Autodesk Inventor part; units mm, degrees
ref_plane "nt_XY" through (0, 0, 0) normal (1, 0, 0) x (0, 0, -1)
ref_plane "nt_YZ" through (0, 0, 0) normal (0, 0, -1) x (0, 1, 0)
ref_plane "nt_ZX" through (0, 0, 0) normal (0, 1, 0) x (1, 0, 0)
sketch "B" plane through (0, 0, 0) normal (1, 0, 0) x (0, 1, 0)
  line L0 (-3.1754, 5.5) -> (-6.3509, 0)
  line L1 (-6.3509, 0) -> (-3.1754, -5.5)
  line L2 (-3.1754, -5.5) -> (3.1754, -5.5)
  line L3 (3.1754, -5.5) -> (6.3509, 0)
  line L4 (6.3509, 0) -> (3.1754, 5.5)
  line L5 (3.1754, 5.5) -> (-3.1754, 5.5)
extrude "Extrusion1" add sketch "B" along normal mid plane 4
sketch "Sketch_2_ALT_Drilling_1" plane through (0, 0, 0) normal (0, 0, 1) x (1, 0, 0)
  line L0 (2, 0) -> (-2, 0)
  line L1 (-2, 0) -> (-2, 4)
  line L2 (-2, 4) -> (-1.4585, 3.4585)
  line L3 (-1.4585, 3.4585) -> (1.4585, 3.4585)
  line L4 (1.4585, 3.4585) -> (2, 4)
  line L5 (2, 4) -> (2, 0)
  line L6 (2, 0) -> (-2, 0)
revolve "Revolution1" cut sketch "Sketch_2_ALT_Drilling_1" angle 360 about axis through (2, 0, 0) along (1, 0, 0)
thread "Thread1"
sketch "Sketch_3" plane through (0, 0, 0) normal (0, 0, 1) x (1, 0, 0)
  line L0 (50, 0) -> (-50, 0)
  line L1 (-7, 1) -> (-2, 1)
  line L2 (-2, 1) -> (-2, 5.5)
  line L3 (-2, 5.5) -> (0, 8.9641)
  line L4 (0, 8.9641) -> (2, 5.5)
  line L5 (2, 5.5) -> (2, 1)
  line L6 (2, 1) -> (7, 1)
  line L7 (7, 1) -> (7, 13.5)
  line L8 (7, 13.5) -> (-7, 13.5)
  line L9 (-7, 13.5) -> (-7, 1)
revolve "Revolution2" cut sketch "Sketch_3" angle 360 about axis through (50, 0, 0) along (1, 0, 0)
ref_plane "nt_XY" through (0, 0, 0) normal (1, 0, 0) x (0, 0, -1)
ref_plane "nt_YZ" through (0, 0, 0) normal (0, 0, -1) x (0, 1, 0)
ref_plane "nt_ZX" through (0, 0, 0) normal (0, 1, 0) x (1, 0, 0)
ref_plane "ntj_XY" through (2, 0, 0) normal (1, 0, 0) x (0, 0, -1)
ref_plane "ntj_YZ" through (2, 0, 0) normal (0, 0, -1) x (0, 1, 0)
ref_plane "ntj_ZX" through (2, 0, 0) normal (0, 1, 0) x (1, 0, 0)
properties part number "SNJ-010C"
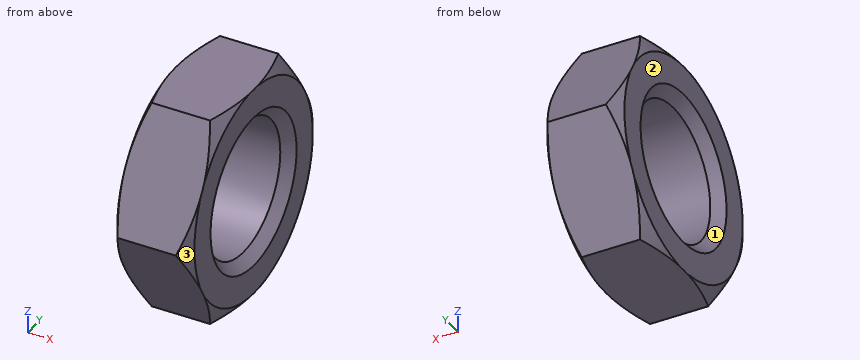
Can you work these out from the model? Positions are in its coordinate system, mm. Face numbers are marked on the shaded views. Round coordinates to 2 decimals unless told otherwise and drop trailing zeros. Order: outer loops, then holes, each group sorted by start corner. A loop starts at its lowest first (then second) coordinate and runs counter-clockwise, first axis right, second up. Notation, with made-up numbers: (26.5, -18.5) -> (38.5, -18.5) arc R22 cw to (38.5, 16.5) -> close; hole circle Ø9 at (3, 38). An arc over 180 degrees is marked (long way). Write each question's results on one line, items separated by ' | '. Start each with the question number.
Item 1: If we section it at A-A, the plane x = 0.45: Write out the boundary of the cut face in (y, z).
Item 2: Please list where these lines run through material, in increasing order: L1, parallel to Z at x = 0.2, y = 0; L2, parallel to Z at x = 0.25, y = -2; L3, parallel to Y at x = 1.7, z = 2.
Item 3: Thinking about a two-plate mould opening in Y: for the marked faces 1, 2 and 3, which applies, +Y half, -Y half, draft (parallel to the pull), parting line (faces both ways), or undercut?
Item 4: Will these pins go through, and if not, where does the flat tip stop? pin 1 (2 mm diameter, centred on x = -1, z = -3.5, fed in from -Y); pin 2 (5 mm diameter, centred on y = 1, z = 3, fed in from -X); pin 3 (1.5 mm diameter, centred on x = 1.5, z = 3, fed in from +Y).
Results:
1) outline: (-6.35, 0) -> (-3.18, -5.5) -> (3.18, -5.5) -> (6.35, 0) -> (3.18, 5.5) -> (-3.18, 5.5) -> close; hole circle Ø6.92 at (0, 0)
2) L1: z = -5.5 to -3.46, 3.46 to 5.5 | L2: z = -5.5 to -2.82, 2.82 to 5.5 | L3: y = -5.2 to -3.11, 3.11 to 5.2
3) face 1: undercut | face 2: draft | face 3: -Y half
4) pin 1: stops at y = -4.91 | pin 2: stops at x = -2 | pin 3: stops at y = 5.05
